Here's the drawing with two shaded views (mm, measured from the low corner). I have some questions. A direction names the side the tool comes from. Round coordinates to 2 decimals unless told otherwise and drop trailing zeros. Write each loop counter-clockwise with the first axis right and the second up, starting at its lowest first coordinate (ties: lowest second). Pieces come first, ordered by that corner, then holes. Notation, with made-up numbers: (14, -40) -> (59, -40) arc R30 ccw to (59, -2) -> close; hole circle Ø9 at (-39, 70.5). An arc over 180 degrees is marked (long way). Use CSV: the item, a comma, the result in double quotes.
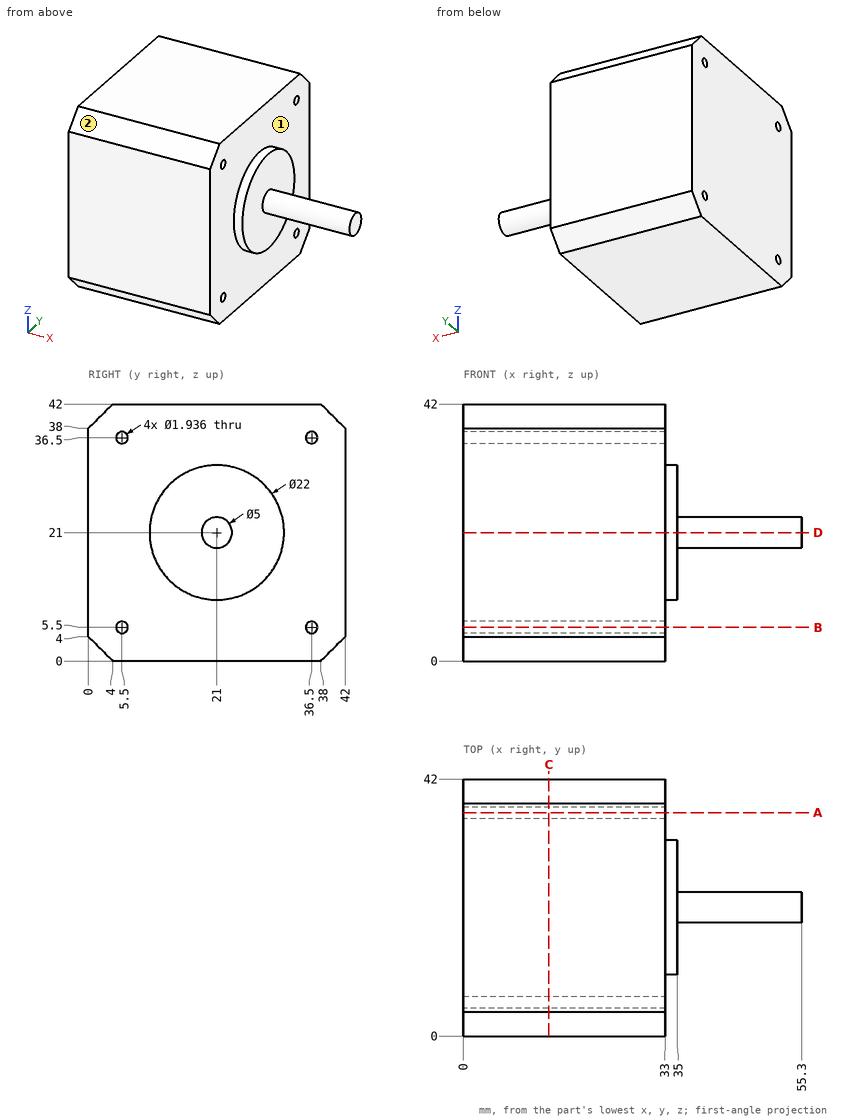
Q1. Please list where these lines run through material, in increasing order: probe 1 along Z at (x, y) = (24.5, 5.5); probe 2 along Z at (x, y) = (9, 5); probe 3 along X at (y, z) = (19, 24).
Resolved:
probe 1,"z = 0 to 4.53, 6.47 to 35.53, 37.47 to 42"
probe 2,"z = 0 to 4.67, 6.33 to 35.67, 37.33 to 42"
probe 3,"x = 0 to 35"
Q2. Suppose I cut it at D-D (z = 21). Write out the boundary of the cut face in (x, y), and give its area (3 significant figures).
Resolved:
outline,"(0, 0) -> (33, 0) -> (33, 10) -> (35, 10) -> (35, 18.5) -> (55.3, 18.5) -> (55.3, 23.5) -> (35, 23.5) -> (35, 32) -> (33, 32) -> (33, 42) -> (0, 42) -> close"
area,"1,530 mm^2"
Q3. Suppose I cut it at C-C (x = 14). Write out the boundary of the cut face in (y, z).
Resolved:
outline,"(0, 4) -> (4, 0) -> (38, 0) -> (42, 4) -> (42, 38) -> (38, 42) -> (4, 42) -> (0, 38) -> close; hole circle Ø1.94 at (5.5, 5.5); hole circle Ø1.94 at (5.5, 36.5); hole circle Ø1.94 at (36.5, 5.5); hole circle Ø1.94 at (36.5, 36.5)"
Q4. Suppose I cut it at A-A (y = 36.5). Write out the boundary of the cut face in (x, z).
Resolved:
outline,"(0, 0) -> (33, 0) -> (33, 4.53) -> (0, 4.53) -> close; (0, 6.47) -> (33, 6.47) -> (33, 35.53) -> (0, 35.53) -> close; (0, 37.47) -> (33, 37.47) -> (33, 42) -> (0, 42) -> close"
Q5. On a 3-axis mill with a long thin cutter (end or side, diameter ignored), from which of +Z, -Z, +X, -X, +Y, -Y can I reach the whole of each face in a straight line? I mean the marked faces 1 and 2. Say none if no direction works.
Resolved:
face 1,"+X"
face 2,"+Z, +X, -X, -Y"
Q6. Will this pin go through, and if not, where does the flat tip stop? P1, Ø3, axis at y = 14.5, z = 34.5, coming from the +X side.
Resolved:
P1,"stops at x = 33"
